Autodesk Inventor part; units mm, degrees
ref_plane "YZ Plane" through (0, 0, 0) normal (1, 0, 0) x (0, 1, 0)
ref_plane "XZ Plane" through (0, 0, 0) normal (0, 1, 0) x (-1, 0, 0)
ref_plane "XY Plane" through (0, 0, 0) normal (0, 0, 1) x (1, 0, 0)
sketch "Skizze1" plane through (0, 0, 0) normal (1, 0, 0) x (0, 1, 0)
  line L0 (0, 0) -> (-10, 0) construction
  circle A0 centre (0, 0) radius 1.1
  circle A1 centre (-10, 0) radius 1.1
  arc A2 (-10, 2.5) -> (-10, -2.5) centre (-10, 0) ccw
  line L1 (-10, -2.5) -> (2.9, -2.5)
  line L2 (-10, 2.5) -> (0.9, 2.5)
  arc A3 (2.9, 0.5) -> (0.9, 2.5) centre (0.9, 0.5) ccw
  line L3 (2.9, 0.5) -> (2.9, -2.5)
  dimension "d0" = 10
  dimension "d1" = 2.2
  dimension "d2" = 2.2
  dimension "d3" = 2.5
  dimension "d8" = 2
  dimension "d9" = 2.9
extrude "Extrusion1" add sketch "Skizze1" along normal mid plane 4
chamfer "Fase1" distance 0.5 angle 45 10 edges at (2, 2.3142, 1.9142) (2, -4.55, 2.5) (2, -12.5, 0) (2, -3.55, -2.5) (2, 2.9, -1) (-2, 2.3142, 1.9142) (-2, -4.55, 2.5) (-2, -12.5, 0) (-2, -3.55, -2.5) (-2, 2.9, -1)
sketch "Skizze4" plane through (-1.5, -10, 2.5) normal (0, 0, 1) x (1, 0, 0)
  line L0 (1.5, 15.98) -> (1.5, -5.58) construction
  line L1 (0, 0) -> (3, 0) construction
  line L2 (0.75, 0.4) -> (2.25, 0.4)
  line L3 (2.25, 0.4) -> (2.25, 0)
  line L4 (2.25, 0) -> (0.75, 0)
  line L5 (0.75, 0) -> (0.75, 0.4)
  line L6 (0.75, 0.4) -> (2.25, 0) construction
  line L7 (2.25, 0.4) -> (0.75, 0) construction
  point P0 (1.5, 10)
  point P1 (1.5, 0.2)
  point P2 (1.5, 0)
  dimension "d23" = 0.4
  dimension "d24" = 1.5
extrude "Extrusion3" cut sketch "Skizze4" against normal blind 0.2
pattern_linear "Rechteckige Anordnung1" count 2 spacing 1 along (0, 1, 0) of "Extrusion3"
equation "\"d2\" = d1"
properties part number "Chipanschlag T1"
Input: part model. Units: mm. Frame: model coordinates. Coordinates: 2 decimals unless noted, no trailing zeros. Loops run counter-clockwise (first coordinate to the right, second up) from the corner with the lowest first, then second, coordinate; pieces in that order, holes last. Notation, with made-up numbers: (-6, 41.5) - (30, 41.5) arc R8 ccw to (30, 53.5) - close; hole circle Ø10 at (-9, -6). An arc over 180 degrees is marked (long way). Answer in a Markdown table with one row per item. Add a question column.
Item 1: Line query: line 1 along Y through (x, z) = (0.4, -0.1); line 2 along Y through (x, z) = (0.35, -1.5); line 3 along Z through (x, y) = (-0.35, 0). Output: solid intervals per line, ascending. Write a range as [from, to].
Item 2: Section query D-D on y = -2.5. Return the cut outline in (x, z).
Item 3: Section query C-C on x = 0.4. Return the cut outline in (y, z), then the cut area to 3 significant figures.
Item 4: Section query A-A on y = 0. Return the cut outline in (x, z).
Item 5: Contact query for a flat-ended pin moving along its axis: P1, Ø1.3, axis at y = -10, z = 0, coming from the +X side. Output: stop coordinate, or through.
Item 6: Mould query, pull axis Z, two halves, no side actions, for faces 1 (the cylindrical face through (-0.028, -8.984, 0.421)), 2 (the conical face through (1.86, -12.14, -0.05)), 3 (the flat face through (0, -5, 2.5)). Classes: released by +Z, released by -Z, zero draft, split by the parting line, or undercut.
Item 7: Section query B-B on z = 0. Return the cut outline in (x, y), then the cut area to 3 significant figures.
Recorded:
| question | item | result |
|---|---|---|
| 1 | line 1 | [-12.5, -11.1], [-8.9, -1.1], [1.1, 2.9] |
| 1 | line 2 | [-12, 2.9] |
| 1 | line 3 | [-2.5, -1.1], [1.1, 2.5] |
| 2 | outline | (-2, -2) - (-1.5, -2.5) - (1.5, -2.5) - (2, -2) - (2, 2) - (1.5, 2.5) - (-1.5, 2.5) - (-2, 2) - close |
| 3 | outline | (-10, -2.5) - (2.9, -2.5) - (2.9, 0.5) arc R2 ccw to (0.9, 2.5) - (-8.6, 2.5) - (-8.6, 2.3) - (-9, 2.3) - (-9, 2.5) - (-9.6, 2.5) - (-9.6, 2.3) - (-10, 2.3) - (-10, 2.5) arc R2.5 ccw to start; hole circle Ø2.2 at (-10, 0); hole circle Ø2.2 at (0, 0) |
| 3 | area | 65.7 mm^2 |
| 4 | outline | (-2, -2) - (-1.5, -2.5) - (1.5, -2.5) - (2, -2) - (2, -1.1) - (-2, -1.1) - close; (-2, 1.1) - (2, 1.1) - (2, 2) - (1.5, 2.5) - (-1.5, 2.5) - (-2, 2) - close |
| 5 | P1 | through |
| 6 | face 1 | undercut |
| 6 | face 2 | split by the parting line |
| 6 | face 3 | released by +Z |
| 7 | outline | (-2, -12) - (-1.5, -12.5) - (1.5, -12.5) - (2, -12) - (2, -11.1) - (-2, -11.1) - close; (-2, -8.9) - (2, -8.9) - (2, -1.1) - (-2, -1.1) - close; (-2, 1.1) - (2, 1.1) - (2, 2.4) - (1.5, 2.9) - (-1.5, 2.9) - (-2, 2.4) - close |
| 7 | area | 43.5 mm^2 |
